Study the drawing (mm; zero at the part's minimum x, y, z) and answer. Round coordinates to 2 decimals unless told otherwise and drop trailing zeros. Order: outer loops, then holes, each group sorted by start corner. A loop starts at its lowest first (then second) coordinate and runs counter-clockwise, first axis right, second up. Notation, with made-up numbers: (-21.5, 1) - (16.5, 1) arc R15 cw to (16.5, 16) - close; hole circle Ø10 at (58.25, -39.5). An arc over 180 degrees is marked (long way). Put each result on its own line as item: value.
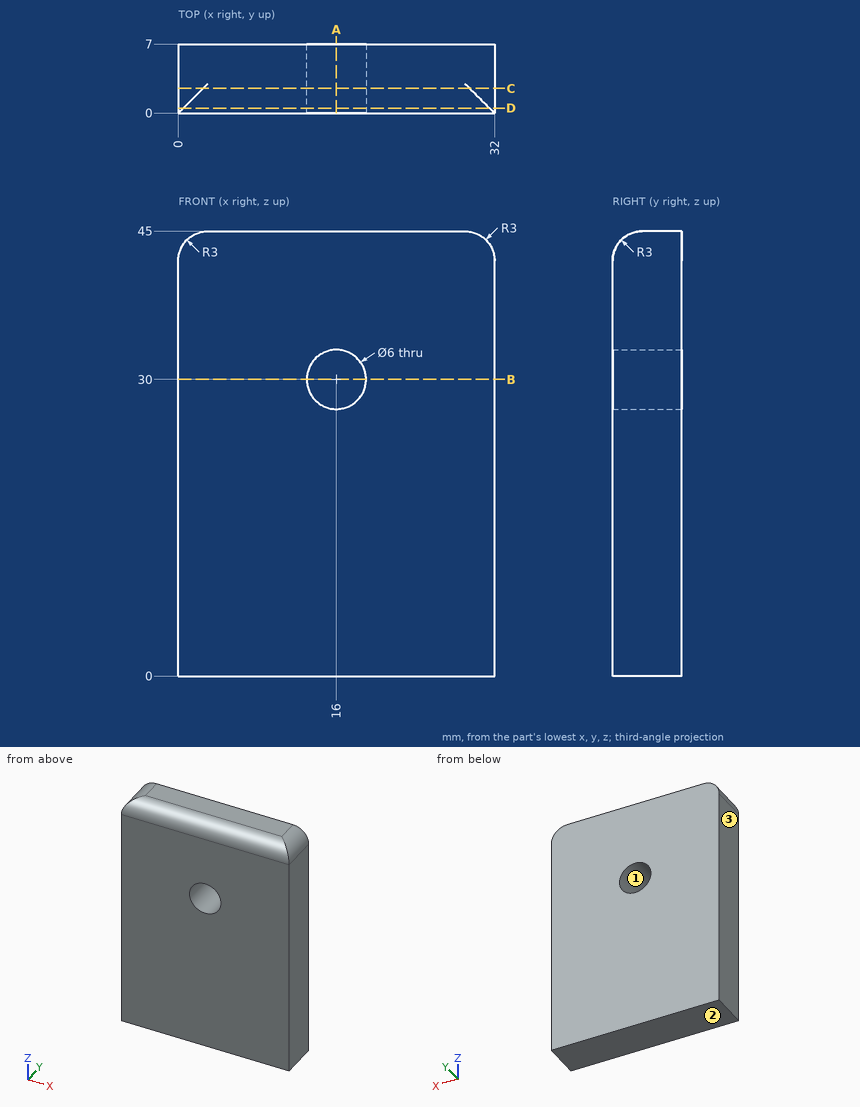
1) Straight lines are drawn through the part: L1, parallel to Z at x = 16, y = 3.75; L2, parallel to Z at x = 16, y = 2; L3, parallel to Z at x = 5.5, y = 2.5. For each, find the intervals that lie inside material, in ascending order. Write a range as from..to.
Findings below:
L1: z = 0..27, 33..45
L2: z = 0..27, 33..44.83
L3: z = 0..44.96
2) A cutting plane is placed at D-D on y = 0.5. Write down the section's boundary in (x, z).
Findings below:
outline: (0, 0) - (32, 0) - (32, 42) arc R3 ccw to (31.5, 43.66) - (0.5, 43.66) arc R3 ccw to (0, 42) - close; hole circle Ø6 at (16, 30)
3) A cutting plane is placed at C-C on y = 2.5. Write down the section's boundary in (x, z), then the cut area to 3 significant figures.
Findings below:
outline: (0, 0) - (32, 0) - (32, 42) arc R3 ccw to (29.5, 44.96) - (2.5, 44.96) arc R3 ccw to (0, 42) - close; hole circle Ø6 at (16, 30)
area: 1,410 mm2
4) A cutting plane is placed at B-B on z = 30. Write down the section's boundary in (x, y), then the cut area to 3 significant figures.
Findings below:
outline: (0, 0) - (13, 0) - (13, 7) - (0, 7) - close; (19, 0) - (32, 0) - (32, 7) - (19, 7) - close
area: 182 mm2
5) For a pull along Z with two mould halves and no side action, classify the marked faces 1, 2 and 3 as pulls with the +Z half, pulls with the -Z half, needs draft (parallel to the pull), parting line crosses it, or undercut.
Findings below:
face 1: undercut
face 2: pulls with the -Z half
face 3: needs draft
6) A cutting plane is placed at A-A on x = 16. Write down the section's boundary in (y, z), then the cut area to 3 significant figures.
Findings below:
outline: (0, 0) - (7, 0) - (7, 27) - (0, 27) - close; (0, 33) - (7, 33) - (7, 45) - (3, 45) arc R3 ccw to (0, 42) - close
area: 271 mm2
